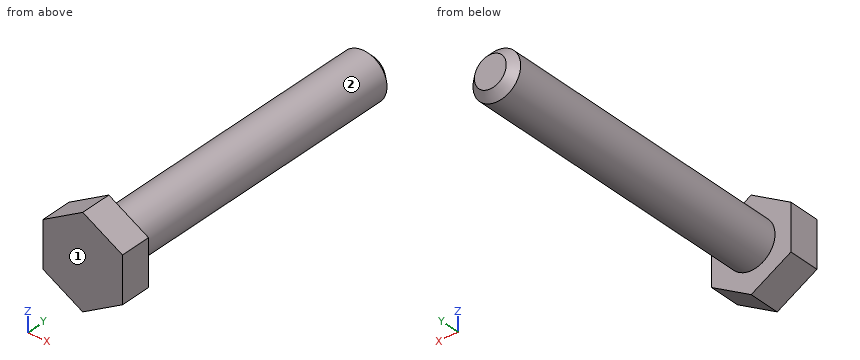
from build123d import *

# Parameters (mm, degrees)
BOSS_EXTRUDE1_DEPTH = 4
SKETCH2_R           = 3
BOSS_EXTRUDE2_DEPTH = 40
CHAMFER1_SIZE       = 1


with BuildPart() as part:
    # Sketch1 → Boss-Extrude1 (new body)
    with BuildSketch(Plane(origin=(0, 0, 0), x_dir=(1, 0, 0), z_dir=(0, 1, 0))):
        Polygon((0, 5.773502692), (-5, 2.886751346), (-5, -2.886751346), (0, -5.773502692), (5, -2.886751346), (5, 2.886751346), align=None)
    extrude(amount=BOSS_EXTRUDE1_DEPTH)

    # Sketch2 → Boss-Extrude2 (add)
    with BuildSketch(Plane(origin=(0, 4, 0), x_dir=(1, 0, 0), z_dir=(0, 1, 0))):
        with Locations(Location((0, 0, 0), (0, 0, 270))):
            Circle(SKETCH2_R)
    extrude(amount=BOSS_EXTRUDE2_DEPTH)

    # Chamfer1
    chamfer1_edges = [part.edges().sort_by_distance(p)[0] for p in [
        (0, 44, -3),
    ]]
    chamfer(chamfer1_edges, length=CHAMFER1_SIZE)


solid = part.part
Geometry: final body of the model. Coordinates: model frame, mm. Face numbers are marked on the shaded views. A direction names the side the tool comes from. Round coordinates to 2 decimals unless told otherwise and drop trailing zeros. Loops run counter-clockwise (first coordinate to the right, second up) from the corner with the lowest first, then second, coordinate; pieces in that order, holes last. Notation, with made-up numbers: M -5,81.25 L 54,81.25 A21 ccw 54,111.25 Z; hole C 89,-35.75 d1. An arc over 180 degrees is marked long. Put each result on its own line as item: value. Start each with the question number.
(1) Section query D-D (z = 4). Return loops of the section in (x, y).
(2) Material intervals for line 1 along Y through (x, z) = (2, 3); line 2 along X through (y, z) = (31, 0); line 3 along X through (y, z) = (35.5, 2.5), sorted ascending. Write a range as [from, to].
(3) Section query C-C (x = -3.5). Return loops of the section in (y, z).
(4) Set-up query: the marked faces 1 and 2. Return all of +Z, -Z, +X, -X, +Y, -Y with unobstructed straight access to the full face (end or side cutting, diameter ignored); none if empty.
(5) Contact query for flat-ended pins moving along their axis: pin 1 Ø1.5 at (x, z) = (1.5, -3.5) entering from +Y; pin 2 Ø1.5 at (x, y) = (3, 34) entering from -Z; pin 3 Ø1.5 at (y, z) = (39, -2.5) entering from +X. Output: stop coordinate, or through.
(6) Section query B-B (y = 26). Return loops of the section in (x, z).
(7) Section query A-A (z = 0). Return loops of the section in (x, y).
Findings below:
1. outline: M -3.07,0 L 3.07,0 L 3.07,4 L -3.07,4 Z
2. line 1: y = [0, 4]
2. line 2: x = [-3, 3]
2. line 3: x = [-1.66, 1.66]
3. outline: M 0,-3.75 L 4,-3.75 L 4,3.75 L 0,3.75 Z
4. face 1: +Z, -Z, +X, -X, -Y
4. face 2: +Y
5. pin 1: stops at y = 4
5. pin 2: stops at z = -1.98
5. pin 3: stops at x = 2.44
6. outline: C 0,0 d6
7. outline: M -5,0 L 5,0 L 5,4 L 3,4 L 3,43 L 2,44 L -2,44 L -3,43 L -3,4 L -5,4 Z
